from build123d import *

# Parameters (mm, degrees)
F0_R     = 8.382
F1_DEPTH = 3.81
F2_W     = 25.4
F2_H     = 3.81
F3_DEPTH = 12.7
F4_R     = 1.397
F5_DEPTH = 25.4
F6_W     = 18.314426
F6_H     = 2.959909
F7_DEPTH = 25.4


with BuildPart() as f1:
    # F0 (on Top) → F1 (new body)
    with BuildSketch(Plane.XY):
        with BuildLine():
            ThreePointArc((25.4, 3.175), (21.680256, 12.155256), (12.7, 15.875))
            Line((12.7, 15.875), (-12.7, 15.875))
            ThreePointArc((-12.7, 15.875), (-21.680256, 12.155256), (-25.4, 3.175))
            Line((-25.4, 3.175), (-25.4, -3.175))
            ThreePointArc((-25.4, -3.175), (-21.680256, -12.155256), (-12.7, -15.875))
            Line((-12.7, -15.875), (12.7, -15.875))
            ThreePointArc((12.7, -15.875), (21.680256, -12.155256), (25.4, -3.175))
            Line((25.4, -3.175), (25.4, 3.175))
        make_face()
        with Locations((-12.7, 3.175)):
            Circle(F0_R, mode=Mode.SUBTRACT)
        with Locations((12.7, 3.175)):
            Circle(F0_R, mode=Mode.SUBTRACT)
    extrude(amount=F1_DEPTH)

    # F2 (on face) → F3 (join)
    with BuildSketch(Plane.XY.offset(3.81)):
        with Locations((0, -13.97)):
            Rectangle(F2_W, F2_H)
    extrude(amount=F3_DEPTH)

    # F4 (on face) → F5 (cut)
    with BuildSketch(Plane(origin=(0, -12.065, 0), x_dir=(-1, 0, 0), z_dir=(0, 1, 0))):
        with Locations((-7.62, 10.16)):
            Circle(F4_R)
        with Locations((7.62, 10.16)):
            Circle(F4_R)
    extrude(amount=-F5_DEPTH, mode=Mode.SUBTRACT)

    # F6 (on face) → F7 (cut)
    with BuildSketch(Plane(origin=(0, 0, 0), x_dir=(1, 0, 0), z_dir=(0, 0, -1))):
        with Locations((0, 8.60223)):
            Rectangle(F6_W, F6_H)
    extrude(amount=-F7_DEPTH, mode=Mode.SUBTRACT)


solid = f1.part
Work out the finished part from the listing and answer in its coordinate system (mm). A direction names the side the tool comes from. Round coordinates to 2 decimals unless told otherwise and drop trailing zeros. Loops run counter-clockwise (first coordinate to the right, second up) from the corner with the lowest first, then second, coordinate; pieces in that order, holes last. Notation, with made-up numbers: (82, -4) - (137, -4) arc R31 ccw to (137, 35) - close; hole circle Ø5 at (-39, 76). An arc over 180 degrees is marked (long way). One line per item, written item: value.
Q1. Find section C-C on y = 0. Give the vertices of the cut face in (x, z).
Check values:
outline: (-25.4, 0) - (-20.46, 0) - (-20.46, 3.81) - (-25.4, 3.81) - close; (-4.94, 0) - (4.94, 0) - (4.94, 3.81) - (-4.94, 3.81) - close; (20.46, 0) - (25.4, 0) - (25.4, 3.81) - (20.46, 3.81) - close
Q2. Straight lines are drawn through the part: probe 1 along X at (y, z) = (6, 1.5); probe 2 along Y at (x, z) = (-6, 2) (3 decimals); probe 3 along Y at (x, z) = (12.7, 1.5) (3 decimals). For each, find the intervals that lie inside material, in ascending order.
Check values:
probe 1: -25.08 to -20.59, -4.81 to 4.81, 20.59 to 25.08
probe 2: -15.875 to -10.082, -7.122 to -1.862, 8.212 to 15.875
probe 3: -15.875 to -5.207, 11.557 to 15.875
Q3. For faces 1 (the flat face through (-9.157, -9, 2)), 2 (the flat face through (25.4, 0, 2)), 3 (the flat face through (12.7, -14, 10)), 4 (the flat face through (0, -12.065, 10)), 5 (the cylindrical face through (7.923, -13.943, 8.796)), determine the directions among +Z, -Z, +X, -X, +Y, -Y from which every point of the face is accessible in a straight line to the end or side of a thin tool.
Check values:
face 1: +Z, -Z
face 2: +Z, -Z, +X, +Y, -Y
face 3: +Z, +X, +Y, -Y
face 4: +Z, +X, -X, +Y
face 5: +Y, -Y
Q4. Find section B-B on x = -7. Give the vertices of the cut face in (y, z) (3 decimals).
Check values:
outline: (-15.875, 0) - (-10.082, 0) - (-10.082, 3.81) - (-12.065, 3.81) - (-12.065, 8.908) - (-15.875, 8.908) - close; (-15.875, 11.412) - (-12.065, 11.412) - (-12.065, 16.51) - (-15.875, 16.51) - close; (-7.122, 0) - (-2.971, 0) - (-2.971, 3.81) - (-7.122, 3.81) - close; (9.321, 0) - (15.875, 0) - (15.875, 3.81) - (9.321, 3.81) - close
Q5. The mould has two halves that part along X. Classify faces 6 (the cylindrical face through (21.778, 12.056, 1.878)), 7 (the cylindrical face through (-13.791, 11.486, 1.878)), 8 (the flat face through (0, -14, 16.51)): +X half, -X half, draft (parallel to the pull), parting line (faces both ways), or undercut.
Check values:
face 6: +X half
face 7: undercut
face 8: draft
Q6. Find section A-A on z = 10.16. Give the vertices of the cut face in (x, y) (3 decimals).
Check values:
outline: (-12.7, -15.875) - (-9.017, -15.875) - (-9.017, -12.065) - (-12.7, -12.065) - close; (-6.223, -15.875) - (6.223, -15.875) - (6.223, -12.065) - (-6.223, -12.065) - close; (9.017, -15.875) - (12.7, -15.875) - (12.7, -12.065) - (9.017, -12.065) - close
Q7. Each of these flat-tipped pins is pushed along its axis until it touches: pin 1 Ø5 at (x, y) = (-1, -6.5) entering from +Z; pin 2 Ø10 at (x, y) = (12.7, 3.175) entering from -Z; pin 3 Ø2.5 at (y, z) = (-8.5, 2) entering from +X; pin 4 Ø1.1 at (y, z) = (-14, 7.5) entering from +X. Where does it stop, or does it pass through?
Check values:
pin 1: z = 3.81
pin 2: through
pin 3: x = 24.73
pin 4: x = 12.7
Q8. Find section D-D on z = 2. Give the vertices of the cut face in (x, y) (3 decimals).
Check values:
outline: (-25.4, -3.175) arc R12.7 ccw to (-12.7, -15.875) - (12.7, -15.875) arc R12.7 ccw to (25.4, -3.175) - (25.4, 3.175) arc R12.7 ccw to (12.7, 15.875) - (-12.7, 15.875) arc R12.7 ccw to (-25.4, 3.175) - close; hole circle Ø16.764 at (-12.7, 3.175); hole (-9.157, -10.082) - (9.157, -10.082) - (9.157, -7.122) - (-9.157, -7.122) - close; hole circle Ø16.764 at (12.7, 3.175)
